Can you work these out from the model? Positions are in its coordinate system, mm. A direction names the side the tool comes from. Coordinates: 2 decimals unless noted, no trailing zeros. Order: outer loops, then holes, each group sorted by start corner. A loop starts at its lowest first (then second) coordinate and runs counter-clockwise, first axis right, second up. Notation, with made-up numbers: M 23.5,-28.5 L 73.5,-28.5 A23 cw 73.5,-4.5 Z; hole C 44.5,20 d9. An arc over 180 degrees is marked long. Answer as CSV lines item,"result". Start each with the question number.
1. Will these pins go through, and if not, where does the flat tip stop? pin 1 (5 mm diameter, centred on y = -9.5, z = 12, fed in from -X); pin 2 (4 mm diameter, centred on x = -4, z = -8, fed in from +Y); pin 3 (2 mm diameter, centred on x = -13.5, z = 14, fed in from -Y); pin 4 (18.5 mm diameter, centred on x = 0, y = 0, fed in from -Z).
2. If we section it at C-C (z = -9): List the corners of the cut face in (x, y) for me, plus the area to 3 significant figures.
3. If we mould it in two halves opening along X, with no side actions, what happens to faces 3 (the face through (-21, -21, 51.347)), 4 (the face through (-2.018, 15.368, -22.676)), 5 (the face through (-13.887, -10.648, -22.183))? For each: released by +X, released by -X, zero draft, split by the parting line, or undercut.
4. I need wall thicknesses on line 1 along Y through (x, z) = (0, -23.25); line 2 along Y through (x, z) = (0, 33); line 3 along X through (y, z) = (13, 44). Which ranges of each line are inside material? Lowest first, please. Write a range as from..to.
5. If we section it at D-D (z = 36): List the corners of the cut face in (x, y) for me.
6. If we section it at A-A (x = 0): List the corners of the cut face in (y, z) for me.
7. On a 3-axis mill with a long thin cutter (end or side, diameter ignored), from which of +Z, -Z, +X, -X, +Y, -Y can I reach the whole of each face in a straight line? I mean faces 1 (the face through (13.38, -25.73, 36.56)), 2 (the face through (-4.036, 30.736, 36.557)). Say none if no direction works.
```python
from build123d import *

# Parameters (mm, degrees)
F0_W    = 2
F0_H    = 30
F2_SIZE = 1


with BuildPart() as f1:
    # F0 (on Front) → F1 (revolve)
    with BuildSketch(Plane.XZ):
        with Locations((30, 36.346545)):
            Rectangle(F0_W, F0_H)
        Polygon((31, 21.346545), (29, 21.346545), (15.5, -7.885725), (17.5, -7.885725), align=None)
        with Locations((16.5, -22.885725)):
            Rectangle(F0_W, F0_H)
    revolve(axis=Axis((0, 0, 12.964369), (0, 0, 1)))

    # F2
    f2_edges = [f1.edges().sort_by_distance(p)[0] for p in [
        (-17.5, 0, -37.885725),
    ]]
    chamfer(f2_edges, length=F2_SIZE)


solid = f1.part
```
Solved:
1,pin 1,"x = -26.43"
1,pin 2,"y = 18.01"
1,pin 3,"y = -24.83"
1,pin 4,"through"
2,outline,"C 0,0 d35; hole C 0,0 d31"
2,area,"207 mm²"
3,face 3,"zero draft"
3,face 4,"undercut"
3,face 5,"split by the parting line"
4,line 1,"-17.5..-15.5, 15.5..17.5"
4,line 2,"-31..-29, 29..31"
4,line 3,"-28.14..-25.92, 25.92..28.14"
5,outline,"C 0,0 d62; hole C 0,0 d58"
6,outline,"M -31,21.35 L -17.5,-7.89 L -17.5,-36.89 L -16.5,-37.89 L -15.5,-37.89 L -15.5,-7.89 L -29,21.35 L -29,51.35 L -31,51.35 Z; M 15.5,-37.89 L 16.5,-37.89 L 17.5,-36.89 L 17.5,-7.89 L 31,21.35 L 31,51.35 L 29,51.35 L 29,21.35 L 15.5,-7.89 Z"
7,face 1,"+Z"
7,face 2,"+Z, -Z"
